```python
from build123d import *

# Parameters (mm, degrees)
SKETCH1_R           = 50
BOSS_EXTRUDE1_DEPTH = 500
SKETCH2_R           = 25
CUT_EXTRUDE1_DEPTH  = 20
SKETCH3_W           = 200
SKETCH3_H           = 400
CUT_EXTRUDE2_DEPTH  = 50


with BuildPart() as part:
    # Sketch1 → Boss-Extrude1 (new body)
    with BuildSketch(Plane(origin=(0, 0, 0), x_dir=(1, 0, 0), z_dir=(0, 1, 0))):
        with Locations(Location((0, 0, 0), (0, 0, 270))):
            Circle(SKETCH1_R)
    extrude(amount=BOSS_EXTRUDE1_DEPTH)

    # Sketch2 → Cut-Extrude1 (cut)
    with BuildSketch(Plane.XZ):
        with Locations(Location((0, 0, 0), (0, 0, 270))):
            Circle(SKETCH2_R)
    extrude(amount=-CUT_EXTRUDE1_DEPTH, mode=Mode.SUBTRACT)

    # Sketch3 → Cut-Extrude2 (cut)
    with BuildSketch(Plane(origin=(30, 0, 0), x_dir=(0, 0, -1), z_dir=(1, 0, 0))):
        with Locations((0, 250)):
            Rectangle(SKETCH3_W, SKETCH3_H)
    extrude(amount=CUT_EXTRUDE2_DEPTH, mode=Mode.SUBTRACT)


solid = part.part
```
Check sheet for the modelled part. Datum: model origin and axes. Units: mm. A direction names the side the tool comes from. Give positions to 0.01 mm unless a question says otherwise; leave off trailing zeros. Loops run counter-clockwise (first coordinate to the right, second up) from the corner with the lowest first, then second, coordinate; pieces in that order, holes last. Notation, with made-up numbers: (85, -13) - (143, -13) arc R11 cw to (143, 1) - close; hole circle Ø3 at (2, -1.5). An arc over 180 degrees is marked (long way). One line per question, with ' | ' between items. Start each with the question number.
1. Cross-section at C-C, the plane y = 139. Enter the section's corners in (x, z), plus the area to 3 significant figures.
2. Material ranges on line 1 along Y through (x, z) = (34.5, 32.5); line 2 along Y through (x, z) = (-10, -20.5); line 3 along X through (y, z) = (15, 0), recorded low to high. Write a range as [from, to].
3. Gauge pin test, flat ends, axial feed: pin 1 Ø1 at (x, y) = (-21, 83) entering from +Z; pin 2 Ø3 at (x, y) = (-33, 247) entering from -Z; pin 3 Ø10 at (y, z) = (252, 7.5) entering from -X. Record the tip position at first contact, or that the pin passes through.
4. Draft check along Y on faces 1 (the flat face through (1, 500, -1)), 2 (the flat face through (30, 253, 1)), 3 (the flat face through (0, 20, 0)), 4 (the flat face through (38, 50, 1)). Enter one of: released by +Y, released by -Y, zero draft, split by the parting line, or undercut.
5. Cross-section at B-B, the plane x = 0. Enter the section's corners in (y, z).
6. Set-up check for faces 5 (the flat face through (22.9, 0, 10.4)), 6 (the cylindrical face through (7.509, 9.86, -23.846)), 7 (the flat face through (38, 450, 1)): record each of +Z, -Z, +X, -X, +Y, -Y from which the full face is reachable in a straight line by a thin tool's end or side.
7. Cross-section at D-D, the plane z = -18.5. Enter the section's corners in (x, y).
8. Cross-section at A-A, the plane z = 0. Enter the section's corners in (x, y), plus the area to 3 significant figures.
Check result:
1) outline: (30, -40) - (30, 40) arc R50 ccw (long way) to start | area: 6,740 mm2
2) line 1: y = [0, 50], [450, 500] | line 2: y = [20, 500] | line 3: x = [-50, -25], [25, 50]
3) pin 1: stops at z = 45.6 | pin 2: stops at z = -38.83 | pin 3: stops at x = -49.94
4) face 1: released by +Y | face 2: undercut | face 3: released by -Y | face 4: undercut
5) outline: (0, -50) - (500, -50) - (500, 50) - (0, 50) - (0, 25) - (20, 25) - (20, -25) - (0, -25) - close
6) face 5: +Z, -Z, +X, -X, -Y | face 6: -Y | face 7: +Z, -Z, +X
7) outline: (-46.45, 0) - (-16.82, 0) - (-16.82, 20) - (16.82, 20) - (16.82, 0) - (46.45, 0) - (46.45, 50) - (30, 50) - (30, 450) - (46.45, 450) - (46.45, 500) - (-46.45, 500) - close
8) outline: (-50, 0) - (-25, 0) - (-25, 20) - (25, 20) - (25, 0) - (50, 0) - (50, 50) - (30, 50) - (30, 450) - (50, 450) - (50, 500) - (-50, 500) - close | area: 41,000 mm2
